Can you work these out from the model? Positions are in its coordinate system, mm. Give positions to 0.01 mm unless a question says otherwise; leave off trailing zeros. Write each loop counter-clockwise with the first axis right and the second up, starting at its lowest first coordinate (ties: lowest second). Pieces come first, ordered by that corner, then holes.
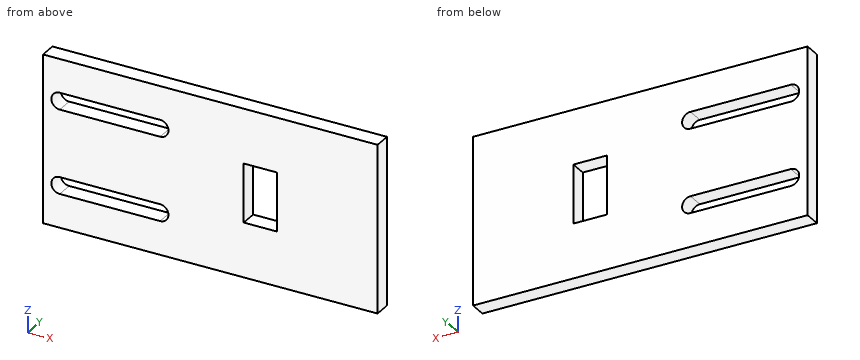
from build123d import *

# Parameters (mm, degrees)
SKETCH2_W           = 100
SKETCH2_H           = 50
BOSS_EXTRUDE1_DEPTH = 5
SKETCH3_W           = 10
SKETCH3_H           = 17.5
CUT_EXTRUDE1_DEPTH  = 7.5
CUT_EXTRUDE2_DEPTH  = 7.5


with BuildPart() as part:
    # Sketch2 → Boss-Extrude1 (new body)
    with BuildSketch(Plane(origin=(0, 0, 0), x_dir=(1, 0, 0), z_dir=(0, 1, 0))):
        Rectangle(SKETCH2_W, SKETCH2_H)
    extrude(amount=BOSS_EXTRUDE1_DEPTH)

    # Sketch3 → Cut-Extrude1 (cut)
    with BuildSketch(Plane(origin=(0, 5, 0), x_dir=(1, 0, 0), z_dir=(0, 1, 0))):
        with Locations((15, 0)):
            Rectangle(SKETCH3_W, SKETCH3_H)
    extrude(amount=-CUT_EXTRUDE1_DEPTH, mode=Mode.SUBTRACT)

    # Sketch4 → Cut-Extrude2 (cut)
    with BuildSketch(Plane(origin=(0, 5, 0), x_dir=(1, 0, 0), z_dir=(0, 1, 0))):
        with BuildLine():
            Line((-45, 15), (-15, 15))
            ThreePointArc((-15, 15), (-12.5, 12.5), (-15, 10))
            Line((-15, 10), (-45, 10))
            ThreePointArc((-45, 10), (-47.5, 12.5), (-45, 15))
        make_face()
        with BuildLine():
            Line((-45, -15), (-15, -15))
            ThreePointArc((-15, -15), (-12.5, -12.5), (-15, -10))
            Line((-15, -10), (-45, -10))
            ThreePointArc((-45, -10), (-47.5, -12.5), (-45, -15))
        make_face()
    extrude(amount=-CUT_EXTRUDE2_DEPTH, mode=Mode.SUBTRACT)


solid = part.part
(1) Imagine slicing it at A-A, the plane x = -20. Write out the boundary of the cut face in (y, z), plus the area to 3 significant figures.
Returned:
outline: (0, -25) - (5, -25) - (5, -15) - (0, -15) - close; (0, -10) - (5, -10) - (5, 10) - (0, 10) - close; (0, 15) - (5, 15) - (5, 25) - (0, 25) - close
area: 200 mm2
(2) If I drill on L1, parallel to Z at x = -24, y = 1.6; L2, parallel to X at y = 2.4, z = -8.5; L3, parallel to Z at x = -46, y = 2.5, over which ranges is the centre line in solid material (lowest first)?
Returned:
L1: z = -25 to -15, -10 to 10, 15 to 25
L2: x = -50 to 10, 20 to 50
L3: z = -25 to -14.79, -10.21 to 10.21, 14.79 to 25
(3) Imagine slicing it at B-B, the plane z = -12.5. Write out the boundary of the cut face in (x, y), plus the area to 3 significant figures.
Returned:
outline: (-50, 0) - (-47.5, 0) - (-47.5, 5) - (-50, 5) - close; (-12.5, 0) - (50, 0) - (50, 5) - (-12.5, 5) - close
area: 325 mm2
(4) Imagine slicing it at C-C, the plane y = 1. Write out the boundary of the cut face in (x, z).
Returned:
outline: (-50, -25) - (50, -25) - (50, 25) - (-50, 25) - close; hole (-45, -15) - (-15, -15) arc R2.5 ccw to (-15, -10) - (-45, -10) arc R2.5 ccw to start; hole (-45, 10) - (-15, 10) arc R2.5 ccw to (-15, 15) - (-45, 15) arc R2.5 ccw to start; hole (10, -8.75) - (20, -8.75) - (20, 8.75) - (10, 8.75) - close
(5) Imagine slicing it at D-D, the plane z = -1. Write out the boundary of the cut face in (x, y).
Returned:
outline: (-50, 0) - (10, 0) - (10, 5) - (-50, 5) - close; (20, 0) - (50, 0) - (50, 5) - (20, 5) - close
